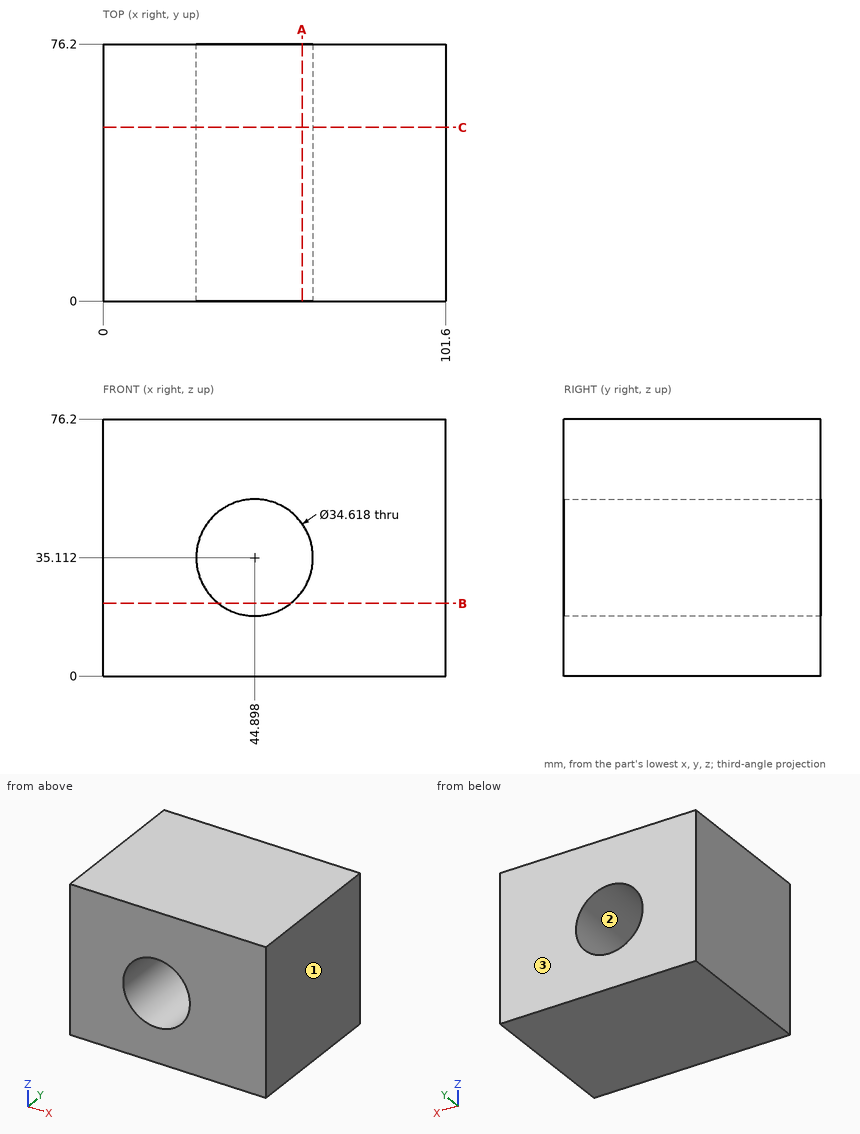
Input: dimensioned drawing with shaded views. Units: mm. Origin: part minimum x, y, z. Give positions to 0.01 mm unless a question says otherwise; leave off trailing zeros. Order: outer loops, then holes, each group sorted by start corner. A loop starts at its lowest first (then second) coordinate and runs counter-clockwise, first axis right, second up. Notation, with made-up numbers: (0, 30.5) -> (33, 30.5) arc R32 cw to (33, 59.5) -> close; hole circle Ø1 at (-6.5, -20.75). An arc over 180 degrees is marked (long way). Use a Markdown table: item, result.
1) Mould query, pull axis X, two halves, no side actions, for the marked faces 1, 2 and 3. Classes: +X half, -X half, draft (parallel to the pull), parting line (faces both ways), or undercut.
Answer list:
| item | result |
|---|---|
| face 1 | +X half |
| face 2 | undercut |
| face 3 | draft |
2) Section query C-C, the plane y = 51.5. Return the cut outline in (x, z), then the cut area to 3 significant figures.
Answer list:
| item | result |
|---|---|
| outline | (0, 0) -> (101.6, 0) -> (101.6, 76.2) -> (0, 76.2) -> close; hole circle Ø34.62 at (44.9, 35.11) |
| area | 6,800 mm² |
3) Section query A-A, the plane x = 59. Return the cut outline in (y, z).
Answer list:
| item | result |
|---|---|
| outline | (0, 0) -> (76.2, 0) -> (76.2, 25.08) -> (0, 25.08) -> close; (0, 45.15) -> (76.2, 45.15) -> (76.2, 76.2) -> (0, 76.2) -> close |
4) Ray query, line 1 along X through (y, z) = (23.5, 44.5) (1 decimal); line 2 along Z through (x, y) = (44, 36.5); line 3 along X through (y, z) = (65.5, 31.5) (1 decimal). Return the intervals inside material, ascending. Write a range as [from, to].
Answer list:
| item | result |
|---|---|
| line 1 | [0, 30.4], [59.4, 101.6] |
| line 2 | [0, 17.83], [52.4, 76.2] |
| line 3 | [0, 28], [61.8, 101.6] |
5) Section query B-B, the plane z = 21.5. Return the cut outline in (x, y), then the cut area to 3 significant figures.
Answer list:
| item | result |
|---|---|
| outline | (0, 0) -> (34.21, 0) -> (34.21, 76.2) -> (0, 76.2) -> close; (55.59, 0) -> (101.6, 0) -> (101.6, 76.2) -> (55.59, 76.2) -> close |
| area | 6,110 mm² |
